Geometry check sheet. Reference: the model listing, model coordinates, mm. A direction names the side the tool comes from. Give positions to 0.01 mm unless a question says otherwise; leave off trailing zeros. Order: outer loops, then holes, each group sorted by start corner. A loop starts at its lowest first (then second) coordinate and runs counter-clockwise, first axis right, second up.
```python
from build123d import *

# Parameters (mm, degrees)
SKETCH1_W                        = 254
SKETCH1_H                        = 3.175
BOSS_EXTRUDE1_DEPTH              = 9.525
BOSS_EXTRUDE2_DEPTH              = 19.05
SKETCH3_R                        = 4.25
CUT_EXTRUDE1_DEPTH               = 129.772942093
SKETCH4_W                        = 9.525
SKETCH4_H                        = 9.525
BOSS_EXTRUDE3_DEPTH              = 4
SKETCH5_R                        = 3
CUT_EXTRUDE2_DEPTH               = 134.81689298
CUT_EXTRUDE2_DRAFT               = 0.5
RIB1_REACH                       = 135.472
SKETCH7_WALL_W                   = 278.469391374
SKETCH7_WALL_H                   = 3.175
MOVE_FACE1_BY                    = 4.572
F_10_24_TAPPED_HOLE1_D           = 4.572
F_10_24_TAPPED_HOLE1_DEPTH       = 9.3335
F_10_24_TAPPED_HOLE1_CSINK_D     = 6.096
F_10_24_TAPPED_HOLE1_CSINK_ANGLE = 90
F_10_24_TAPPED_HOLE1_TIP         = 1.373567375
F_4_40_TAPPED_HOLE1_D            = 2.667
F_4_40_TAPPED_HOLE1_DEPTH        = 9.129125
F_4_40_TAPPED_HOLE1_CSINK_D      = 4.1148
F_4_40_TAPPED_HOLE1_CSINK_ANGLE  = 90
F_4_40_TAPPED_HOLE1_TIP          = 0.801247635
CHAMFER1_SIZE                    = 1.5875


with BuildPart() as part:
    # Sketch1 → Boss-Extrude1 (new body)
    with BuildSketch(Plane(origin=(0, 0, 0), x_dir=(1, 0, 0), z_dir=(0, 1, 0))):
        Rectangle(SKETCH1_W, SKETCH1_H)
    extrude(amount=BOSS_EXTRUDE1_DEPTH)

    # Sketch2 → Boss-Extrude2 (add)
    with BuildSketch(Plane(origin=(0, 0, 0), x_dir=(1, 0, 0), z_dir=(0, 1, 0))):
        with BuildLine():
            Line((126.603125, 9.516728179), (126.603125, -9.516728179))
            ThreePointArc((126.603125, -9.516728179), (117.475, 0), (126.603125, 9.516728179))
        make_face()
    extrude(amount=BOSS_EXTRUDE2_DEPTH)

    # Sketch3 → Cut-Extrude1 (cut, through all)
    with BuildSketch(Plane(origin=(0, 19.05, 0), x_dir=(1, 0, 0), z_dir=(0, 1, 0))):
        with Locations((127, 0)):
            Circle(SKETCH3_R)
    extrude(amount=-CUT_EXTRUDE1_DEPTH, mode=Mode.SUBTRACT)

    # Sketch4 → Boss-Extrude3 (add, symmetric)
    with BuildSketch(Plane.XY):
        with Locations((-127, 4.7625)):
            Rectangle(SKETCH4_W, SKETCH4_H)
    extrude(amount=BOSS_EXTRUDE3_DEPTH, both=True)


with BuildPart() as cut_extrude2_tool:
    # Sketch5 → Cut-Extrude2 (with draft: the straight prism first)
    with BuildSketch(Plane.XY.offset(4)):
        with Locations((-127, 4.7625)):
            Circle(SKETCH5_R)
    extrude(amount=-CUT_EXTRUDE2_DEPTH)
    # Cut-Extrude2: the draft: its side faces are tilted about the plane it starts from
    cut_extrude2_sides = [cut_extrude2_tool.faces().sort_by_distance(p)[0] for p in [
        (-130, 4.7625, -63.40844649),
    ]]
    draft(cut_extrude2_sides, Plane.XY.offset(4), CUT_EXTRUDE2_DRAFT)


with BuildPart() as part_1:
    add(part.part)

    # Cut-Extrude2: cut by cut_extrude2_tool
    add(cut_extrude2_tool.part, mode=Mode.SUBTRACT)

    # Sketch7 wall → Rib1 (add, up to next)
    with BuildSketch(Plane(origin=(114.107403955, 12.892596045, 0), x_dir=(0.707106781187, 0.707106781187, 0), z_dir=(-0.707106781187, 0.707106781187, 0)), mode=Mode.PRIVATE) as rib1_sk1:
        Rectangle(SKETCH7_WALL_W, SKETCH7_WALL_H)
    rib1_tool1 = extrude(rib1_sk1.sketch, amount=-RIB1_REACH, mode=Mode.PRIVATE) - part_1.part
    add(rib1_tool1.solids().sort_by_distance((114.107403955, 12.892596045, 0))[0])

    # Move Face1: a face moved outward by 4.572
    extrude(part_1.faces().sort_by_distance((-131.7625, 4.7625, 0))[0], amount=MOVE_FACE1_BY, dir=(-1, 0, 0))

    # #10-24 Tapped Hole1
    with Locations(Plane.ZY.offset(136.3345)):
        with Locations((0, 4.7625)):
            CounterSinkHole(F_10_24_TAPPED_HOLE1_D / 2, F_10_24_TAPPED_HOLE1_CSINK_D / 2, depth=F_10_24_TAPPED_HOLE1_DEPTH, counter_sink_angle=F_10_24_TAPPED_HOLE1_CSINK_ANGLE)
            with Locations((0, 0, -(F_10_24_TAPPED_HOLE1_DEPTH + F_10_24_TAPPED_HOLE1_TIP / 2))):  # 118° drill point
                Cone(0, F_10_24_TAPPED_HOLE1_D / 2, F_10_24_TAPPED_HOLE1_TIP, mode=Mode.SUBTRACT)

    # #4-40 Tapped Hole1
    with Locations(Plane(origin=(126.603125, 0, 0), x_dir=(0, 0, -1), z_dir=(1, 0, 0))):
        with Locations((-6.874078522, 9.525), (6.874078522, 9.525)):
            CounterSinkHole(F_4_40_TAPPED_HOLE1_D / 2, F_4_40_TAPPED_HOLE1_CSINK_D / 2, depth=F_4_40_TAPPED_HOLE1_DEPTH, counter_sink_angle=F_4_40_TAPPED_HOLE1_CSINK_ANGLE)
            with Locations((0, 0, -(F_4_40_TAPPED_HOLE1_DEPTH + F_4_40_TAPPED_HOLE1_TIP / 2))):  # 118° drill point
                Cone(0, F_4_40_TAPPED_HOLE1_D / 2, F_4_40_TAPPED_HOLE1_TIP, mode=Mode.SUBTRACT)

    # Chamfer1
    # the kernel refuses this chamfer: 1.93751941, 1.5875 mm, written as the material it adds along each edge
    with BuildSketch(Plane(origin=(117.608223344, 0, -1.5875), x_dir=(-1, 0, 0), z_dir=(0, 1, 0))) as chamfer1_piece_1_section:
        with BuildLine():
            Line((CHAMFER1_SIZE, 0), (-0.683137079, -2.270637079))
            ThreePointArc((-0.683137079, -2.270637079), (-0.280625297, -1.189647084), (0, 0))
            Line((0, 0), (CHAMFER1_SIZE, 0))
        make_face()
    chamfer1_piece_1 = extrude(amount=22.492706814, mode=Mode.PRIVATE)
    chamfer1_piece_1 = split(chamfer1_piece_1, bisect_by=Plane(origin=(109.411515627, 8.196707717, -1.5875), z_dir=(0.7071067811865476, -0.7071067811865476, 0)), keep=Keep.TOP, mode=Mode.PRIVATE)
    add(chamfer1_piece_1)
    with BuildSketch(Plane(origin=(117.608223344, 22.492706814, 1.5875), x_dir=(-1, 0, 0), z_dir=(0, -1, 0))) as chamfer1_piece_2_section:
        with BuildLine():
            Line((CHAMFER1_SIZE, 0), (-0.683137079, -2.270637079))
            ThreePointArc((-0.683137079, -2.270637079), (-0.280625297, -1.189647084), (0, 0))
            Line((0, 0), (CHAMFER1_SIZE, 0))
        make_face()
    chamfer1_piece_2 = extrude(amount=22.492706814, mode=Mode.PRIVATE)
    chamfer1_piece_2 = split(chamfer1_piece_2, bisect_by=Plane(origin=(120.657869034, 19.443061124, 1.5875), z_dir=(0.7071067811865476, -0.7071067811865476, 0)), keep=Keep.TOP, mode=Mode.PRIVATE)
    add(chamfer1_piece_2)
    # the kernel refuses this chamfer: 1.93751941, 1.5875 mm, written as the material it takes off along each edge
    with BuildSketch(Plane(origin=(-122.2375, -4.082546743, -4), x_dir=(0, 0, 1), z_dir=(0, 1, 0)), Plane(origin=(-122.2375, -4.082546743, 4), x_dir=(-1, 0, 0), z_dir=(0, 1, 0))) as chamfer1_2_piece_1:
        Polygon((CHAMFER1_SIZE, 0), (0, -CHAMFER1_SIZE), (0, 0), align=None)
    extrude(amount=17.690093487, mode=Mode.SUBTRACT)
    with BuildSketch(Plane(origin=(-136.3345, 13.607546743, -4), x_dir=(1, 0, 0), z_dir=(0, -1, 0)), Plane(origin=(-136.3345, 13.607546743, 4), x_dir=(0, 0, -1), z_dir=(0, -1, 0))) as chamfer1_2_piece_2:
        Polygon((CHAMFER1_SIZE, 0), (0, CHAMFER1_SIZE), (0, 0), align=None)
    extrude(amount=17.690093487, mode=Mode.SUBTRACT)


solid = part_1.part
```
Q1. Access from +Z, -Z, +X, -X, +Y, -Y to the whole of each face (thin tool, end or side, straight path). Record for faces 1 (the face through (-130.4, 4.7, -4)), 2 (the face through (126.603, 7, 7)), 3 (the face through (122, 19.05, 0)), 4 (the face through (-21, 9.525, 0)), 5 (the face through (-130.4, 4.7, 4)).
Q2. Cross-section at A-A, the plane x = -41. Record the boundary of the cut face in (y, z) (1 decimal), and give its area (3 significant figures).
Q3. Release check for a two-part mould opening along Z. For faces 6 (the face through (-132.24, 2.53, 0.5)), 7 (the face through (-2, 6, -1.588)), 8 (the face through (-2, 6, 1.588)) record: pulls with the +Z half, pulls with the -Z half, needs draft (parallel to the pull), parting line crosses it, or undercut.
Q4. Gauge pin test, flat ends, axial feed: P1, Ø2, axis at y = 12.5, z = -1, coming from the -X side; P2, Ø10.5, axis at x = -130, y = 7, coming from the +Z side; P3, Ø7.5, axis at x = -2.5, y = 6.5, coming from the +Z side. Record the tip position at first contact, or that the pin passes through.
Q5. Thickness scan on L1, parallel to X at y = 7.5, z = -3 (3 decimals); L2, parallel to Y at x = -133.75, z = 0 (1 decimal); L3, parallel to Y at x = 55, z = 1.5 (3 decimals). Record the ranges inside material, lowest first.
Answers follow:
1. face 1: -Z, -X, +Y, -Y
1. face 2: +Z, -Z, +X, +Y, -Y
1. face 3: +Z, -Z, +X, -X, +Y
1. face 4: +Z, -Z, -X, +Y
1. face 5: +Z, -X, +Y, -Y
2. outline: (0, -1.6) - (9.5, -1.6) - (9.5, 1.6) - (0, 1.6) - close
2. area: 30.2 mm2
3. face 6: undercut
3. face 7: pulls with the -Z half
3. face 8: pulls with the +Z half
4. P1: stops at x = 112.71
4. P2: stops at z = 4
4. P3: stops at z = 1.59
5. L1: x = -135.747 to -128.37, -125.63 to -122.825, 117.433 to 123.99
5. L2: y = 0 to 2.5, 7 to 9.5
5. L3: y = 0 to 9.525
